Read the model definition and answer for the solid it produces. Units are mm, in the model's axes. A direction names the side the tool comes from. Give positions to 0.01 mm unless a question says otherwise; leave off trailing zeros. Loops run counter-clockwise (first coordinate to the right, second up) from the corner with the lowest first, then second, coordinate; pieces in that order, holes last. Notation, with made-up numbers: M -15,-38.75 L 26,-38.75 A11 ccw 26,-24.75 Z; hole C -11,4 d8. An arc over 180 degrees is marked long. Return JSON: item names as keys, results as strings. Group by question number.
```python
from build123d import *

# Parameters (mm, degrees)
F0_W     = 550
F0_H     = 595
F1_DEPTH = 5
F0_H_2   = 270
F2_DEPTH = 5
F0_H_3   = 135
F3_DEPTH = 5


with BuildPart() as f1:
    # F0 (on Right) → F1 (new body)
    with BuildSketch(Plane.YZ):
        with Locations((-4.257952, 67.584985)):
            Rectangle(F0_W, F0_H)
        with BuildLine():
            ThreePointArc((-229.257952, 275.084985), (-217.542223, 303.369257), (-189.257952, 315.084985))
            Line((-189.257952, 315.084985), (-4.257952, 315.084985))
            Line((-4.257952, 315.084985), (180.742048, 315.084985))
            ThreePointArc((180.742048, 315.084985), (209.026319, 303.369257), (220.742048, 275.084985))
            Line((220.742048, 275.084985), (220.742048, 67.584985))
            Line((220.742048, 67.584985), (220.742048, -139.915015))
            ThreePointArc((220.742048, -139.915015), (209.026319, -168.199286), (180.742048, -179.915015))
            Line((180.742048, -179.915015), (-4.257952, -179.915015))
            Line((-4.257952, -179.915015), (-189.257952, -179.915015))
            ThreePointArc((-189.257952, -179.915015), (-217.542223, -168.199286), (-229.257952, -139.915015))
            Line((-229.257952, -139.915015), (-229.257952, 67.584985))
            Line((-229.257952, 67.584985), (-229.257952, 275.084985))
        make_face(mode=Mode.SUBTRACT)
    extrude(amount=F1_DEPTH)

    # F0 (on Right) → F2 (join)
    with BuildSketch(Plane.YZ):
        with Locations((-4.257952, 500.084985)):
            Rectangle(F0_W, F0_H_2)
    extrude(amount=F2_DEPTH)

    # F0 (on Right) → F3 (join)
    with BuildSketch(Plane.YZ):
        with Locations((-4.257952, -297.415015)):
            Rectangle(F0_W, F0_H_3)
    extrude(amount=F3_DEPTH)


solid = f1.part
```
1. Find section C-C (x = 3.4). Write down the section's boundary in (y, z), and give its area (3 significant figures).
2. The mould has two halves that part along Z. Classify faces 1 (the cylindrical face through (2.46, -217.85, 303.06)), 2 (the flat face through (5, -8, 364)): +Z half, -Z half, draft (parallel to the pull), parting line (faces both ways), or undercut.
3. Find section A-A (z = 203.5). Write down the section's boundary in (x, y).
4. Find section B-B (y = -135). Write down the section's boundary in (x, z).
5. For faces 3 (the flat face through (0, -8, 364)), 4 (the cylindrical face through (2.46, 208.71, 303.68)), determine the directions among +Z, -Z, +X, -X, +Y, -Y from which every point of the face is accessible in a straight line to the end or side of a thin tool.
6. Straight lines are drawn through the part: line 1 along Z through (x, y) = (3.25, 156.5); line 2 along Y through (x, z) = (0.35, 27.5); line 3 along Y through (x, z) = (0.6, 291.5). For each, find the intervals that lie inside material, in ascending order.
Result:
{
 "1": {"outline": "M -279.26,-364.92 L 270.74,-364.92 L 270.74,635.08 L -279.26,635.08 Z; hole M -229.26,-139.92 A40 ccw -189.26,-179.92 L 180.74,-179.92 A40 ccw 220.74,-139.92 L 220.74,275.08 A40 ccw 180.74,315.08 L -189.26,315.08 A40 ccw -229.26,275.08 Z", "area": "329,000 mm2"},
 "2": {"face 1": "undercut", "face 2": "draft"},
 "3": {"outline": "M 0,-279.26 L 5,-279.26 L 5,-229.26 L 0,-229.26 Z; M 0,220.74 L 5,220.74 L 5,270.74 L 0,270.74 Z"},
 "4": {"outline": "M 0,-364.92 L 5,-364.92 L 5,-179.92 L 0,-179.92 Z; M 0,315.08 L 5,315.08 L 5,635.08 L 0,635.08 Z"},
 "5": {"face 3": "+Z, -Z, -X, +Y, -Y", "face 4": "+X, -X"},
 "6": {"line 1": "z = -364.92 to -179.92, 315.08 to 635.08", "line 2": "y = -279.26 to -229.26, 220.74 to 270.74", "line 3": "y = -279.26 to -225.73, 217.22 to 270.74"}
}
